Can you work these out from the model? Positions are in its coordinate system, mm. A direction names the side the tool comes from. Round coordinates to 2 decimals unless told otherwise and drop trailing zeros. Loops run counter-clockwise (first coordinate to the right, second up) from the corner with the lowest first, then second, coordinate; pieces in that order, holes last.
from build123d import *

# Parameters (mm, degrees)
SKETCH_1_W          = 24.5
SKETCH_1_H          = 3.1
EXTRUDE_1_DEPTH     = 3
FILLET_1_R          = 1
EXTRUDE_START       = -3.1
SKETCH_2_W          = 6
SKETCH_2_H          = 4.4
EXTRUDE_2_DEPTH     = 10.8
CUT_EXTRUDE_1_REACH = 16.777
SKETCH_2_3_R        = 1.65
CHAMFER_1_SIZE      = 1
SKETCH_3_W          = 1
SKETCH_3_H          = 1
CUT_EXTRUDE_2_DEPTH = 3.8
SKETCH_4_R          = 0.2
EXTRUDE_3_DEPTH     = 2.2


with BuildPart() as part:
    # Эскиз1 → Бобышка-Вытянуть1 (new, symmetric)
    with BuildSketch(Plane(origin=(0, 0, 0), x_dir=(0, 0, -1), z_dir=(1, 0, 0))):
        Rectangle(SKETCH_1_W, SKETCH_1_H)
    extrude(amount=EXTRUDE_1_DEPTH, both=True)

    # Скругление1
    fillet_1_edges = [part.edges().sort_by_distance(p)[0] for p in [
        (3, 0, 12.25),
        (-3, 0, 12.25),
        (-3, 0, -12.25),
        (3, 0, -12.25),
    ]]
    fillet(fillet_1_edges, radius=FILLET_1_R)

    # Эскиз2 → Бобышка-Вытянуть2 (add)
    with BuildSketch(Plane(origin=(0, 1.55, 0), x_dir=(1, 0, 0), z_dir=(0, 1, 0)).offset(EXTRUDE_START)):
        with Locations((0, 3.75)):
            Rectangle(SKETCH_2_W, SKETCH_2_H)
        with Locations((0, -3.75)):
            Rectangle(SKETCH_2_W, SKETCH_2_H)
    extrude(amount=EXTRUDE_2_DEPTH)

    # Эскиз2<3> → Вырез-Вытянуть1 (cut, up to next)
    with BuildSketch(Plane(origin=(0, 1.55, 0), x_dir=(1, 0, 0), z_dir=(0, 1, 0)), mode=Mode.PRIVATE) as cut_extrude_1_sk1:
        with Locations(Location((0, -9.5, 0), (0, 0, 270))):
            Circle(SKETCH_2_3_R)
    cut_extrude_1_tool1 = extrude(cut_extrude_1_sk1.sketch, amount=-CUT_EXTRUDE_1_REACH, mode=Mode.PRIVATE) & part.part
    # Эскиз2<3> → Вырез-Вытянуть1 (cut, up to next)
    with BuildSketch(Plane(origin=(0, 1.55, 0), x_dir=(1, 0, 0), z_dir=(0, 1, 0)), mode=Mode.PRIVATE) as cut_extrude_1_sk2:
        with Locations(Location((0, 9.5, 0), (0, 0, 270))):
            Circle(SKETCH_2_3_R)
    cut_extrude_1_tool2 = extrude(cut_extrude_1_sk2.sketch, amount=-CUT_EXTRUDE_1_REACH, mode=Mode.PRIVATE) & part.part
    add(cut_extrude_1_tool1.solids().sort_by_distance((0, 1.55, 9.5))[0], mode=Mode.SUBTRACT)
    add(cut_extrude_1_tool2.solids().sort_by_distance((0, 1.55, -9.5))[0], mode=Mode.SUBTRACT)

    # Фаска1
    chamfer_1_edges = [part.edges().sort_by_distance(p)[0] for p in [
        (0, 9.25, 5.95),
    ]]
    chamfer(chamfer_1_edges, length=CHAMFER_1_SIZE)

    # Эскиз3 → Вырез-Вытянуть2 (cut)
    with BuildSketch(Plane(origin=(0, 9.25, 0), x_dir=(1, 0, 0), z_dir=(0, 1, 0))):
        with Locations((0, 2.05)):
            Rectangle(SKETCH_3_W, SKETCH_3_H)
        with Locations((0, -2.05)):
            Rectangle(SKETCH_3_W, SKETCH_3_H)
    extrude(amount=-CUT_EXTRUDE_2_DEPTH, mode=Mode.SUBTRACT)

    # Эскиз4 → Бобышка-Вытянуть3 (add)
    with BuildSketch(Plane.XZ.offset(1.55)):
        with Locations(Location((-1.27, 3.8, 0), (0, 0, 90))):
            Circle(SKETCH_4_R)
        with Locations(Location((1.27, 3.8, 0), (0, 0, 90))):
            Circle(SKETCH_4_R)
        with Locations(Location((1.27, -3.8, 0), (0, 0, 90))):
            Circle(SKETCH_4_R)
        with Locations(Location((-1.27, -3.8, 0), (0, 0, 90))):
            Circle(SKETCH_4_R)
    extrude(amount=EXTRUDE_3_DEPTH)


solid = part.part
(1) For faces 1 (the flat face through (0, 5, 5.95)), 2 (the flat face through (0, 5, 1.55)), 3 (the flat face through (0, 5.45, 2)), 4 (the flat face through (0, 0, 12.25)), which set-ups out of +Z, -Z, +X, -X, +Y, -Y let a thin tool reach every point of the face, with its end or its side?
Worked answers:
face 1: +Z, +X, -X, +Y
face 2: +X, -X, +Y
face 3: +Y
face 4: +Z, +X, -X, +Y, -Y
(2) If we section it at B-B, the plane z = 9.5: List the corners of the cut face in (x, y) for me, then the cut area to 3 significant figures.
Worked answers:
outline: (-3, -1.55) - (-1.65, -1.55) - (-1.65, 1.55) - (-3, 1.55) - close; (1.65, -1.55) - (3, -1.55) - (3, 1.55) - (1.65, 1.55) - close
area: 8.37 mm2
(3) If I drill on line 1 (Z direction, x = -0.4, y = 3.75); line 2 (X direction, y = -0.9, z = -9.5); line 3 (Z direction, x = 1.5, y = 0), over which ranges is the centre line in solid material (lowest first)?
Worked answers:
line 1: z = -5.95 to -1.55, 1.55 to 5.95
line 2: x = -3 to -1.65, 1.65 to 3
line 3: z = -12.25 to -10.19, -8.81 to 8.81, 10.19 to 12.25
(4) If we mould it in two halves opening along Z, with no side actions, what happens to faces 5 (the flat face through (0, 5, -5.95)), 6 (the flat face through (0.5, 7, -2)), 7 (the flat face through (0.5, 7, 2)), 8 (the cylindrical face through (2.699, 0.022, 11.965))? For each: released by +Z, released by -Z, zero draft, split by the parting line, or undercut.
Worked answers:
face 5: released by -Z
face 6: undercut
face 7: undercut
face 8: released by +Z
(5) If we section it at A-A, the plane y = 6: List the corners of the cut face in (x, z) for me, then the cut area to 3 significant figures.
Worked answers:
outline: (-3, -5.95) - (3, -5.95) - (3, -1.55) - (0.5, -1.55) - (0.5, -2.55) - (-0.5, -2.55) - (-0.5, -1.55) - (-3, -1.55) - close; (-3, 1.55) - (-0.5, 1.55) - (-0.5, 2.55) - (0.5, 2.55) - (0.5, 1.55) - (3, 1.55) - (3, 5.95) - (-3, 5.95) - close
area: 50.8 mm2
(6) Will these pins go through, and if not, where does the flat tip stop? P1, Ø3, axis at x = -2, y = 5.5, coming from the -Z side; P2, Ø3, axis at x = 0.5, z = -10.5, coming from the +Y side; P3, Ø3, axis at x = -0.5, z = -2, coming from the -Y side; P4, Ø1.8, axis at x = 0, z = 10, coming from the +Y side.
Worked answers:
P1: stops at z = -5.95
P2: stops at y = 1.55
P3: stops at y = -1.55
P4: passes through
(7) If we section it at D-D, the plane x = -2.6: List the corners of the cut face in (y, z) for me.
Worked answers:
outline: (-1.55, -12.05) - (1.55, -12.05) - (1.55, -5.95) - (9.25, -5.95) - (9.25, -1.55) - (1.55, -1.55) - (1.55, 1.55) - (9.25, 1.55) - (9.25, 4.95) - (8.25, 5.95) - (1.55, 5.95) - (1.55, 12.05) - (-1.55, 12.05) - close
(8) If we section it at C-C, the plane z = -2.25: List the corners of the cut face in (x, y) for me, then the cut area to 3 significant figures.
Worked answers:
outline: (-3, -1.55) - (3, -1.55) - (3, 9.25) - (0.5, 9.25) - (0.5, 5.45) - (-0.5, 5.45) - (-0.5, 9.25) - (-3, 9.25) - close
area: 61.0 mm2
